Geometry check sheet. Reference: the model listing, model coordinates, mm. Round coordinates to 2 decimals unless told otherwise and drop trailing zeros. Loops run counter-clockwise (first coordinate to the right, second up) from the corner with the lowest first, then second, coordinate; pieces in that order, holes last. Notation, with made-up numbers: (-30.5, 35) -> (-15.5, 35) arc R20 cw to (-15.5, 55) -> close; hole circle Ø3 at (11.25, 6.5). An arc over 180 degrees is marked (long way). Use a Markdown table: item, result. Add a question column.
Q1. Gauge pin test, flat ends, axial feed: P1, Ø3, axis at y = -2, z = 9, coming from the -X side; P2, Ø2, axis at x = -2.5, y = -2.5, coming from the -Z side; P3, Ø1.5, axis at x = -2.5, y = -1, coming from the -Z side. Record the tip position at first contact, or that the pin passes through.
Q2. Sectioned sample at D-D, the plane x = 2.75. Enter the section's corners in (y, z).
Q3. Release check for a two-part mould opening along Z. For faces 1 (the face through (2.76, -2.46, 19.47)), 2 (the face through (0, 0, 19)), 3 (the face through (-1.5, -2.46, 0.07)) record: released by +Z, released by -Z, zero draft, split by the parting line, or undercut.
Q4. Sectioned sample at C-C, the plane z = 1. Enter the section's corners in (x, y), then the cut area to 3 significant figures.
Q5. Sectioned sample at B-B, the plane y = -4. Enter the section's corners in (x, z), then the cut area to 3 significant figures.
Q6. Material ranges on L1, parallel to Z at x = 0, y = -2.75; L2, parallel to Z at x = -1, y = -2.8; L3, parallel to X at y = -4.2, z = 3, recorded low to high.
Q7. Sectioned sample at A-A, the plane x = -0.5. Enter the section's corners in (y, z), then the cut area to 3 significant figures.
```python
from build123d import *

# Parameters (mm, degrees)
F0_R     = 1.5
F1_DEPTH = 5


with BuildPart() as f1:
    # F0 (on Front) → F1 (new body)
    with BuildSketch(Plane.XZ):
        with BuildLine():
            Line((-2, 39.5), (-3.5, 0))
            ThreePointArc((-3.5, 0), (-2.474874, -2.474874), (0, -3.5))
            ThreePointArc((0, -3.5), (2.474874, -2.474874), (3.5, 0))
            Line((3.5, 0), (2, 39.5))
            ThreePointArc((2, 39.5), (1.414214, 40.914214), (0, 41.5))
            ThreePointArc((0, 41.5), (-1.414214, 40.914214), (-2, 39.5))
        make_face()
        Circle(F0_R, mode=Mode.SUBTRACT)
    extrude(amount=F1_DEPTH)


solid = f1.part
```
Values:
| question | item | result |
|---|---|---|
| 1 | P1 | x = -3.22 |
| 1 | P2 | z = -3.16 |
| 1 | P3 | z = -3.03 |
| 2 | outline | (-5, -2.17) -> (0, -2.17) -> (0, 19.75) -> (-5, 19.75) -> close |
| 3 | face 1 | released by +Z |
| 3 | face 2 | zero draft |
| 3 | face 3 | undercut |
| 4 | outline | (-3.46, -5) -> (-1.12, -5) -> (-1.12, 0) -> (-3.46, 0) -> close; (1.12, -5) -> (3.46, -5) -> (3.46, 0) -> (1.12, 0) -> close |
| 4 | area | 23.4 mm^2 |
| 5 | outline | (-3.5, 0) arc R3.5 ccw to (0, -3.5) arc R3.5 ccw to (3.5, 0) -> (2, 39.5) arc R2 ccw to (0, 41.5) arc R2 ccw to (-2, 39.5) -> close; hole circle Ø3 at (0, 0) |
| 5 | area | 236 mm^2 |
| 6 | L1 | -3.5 to -1.5, 1.5 to 41.5 |
| 6 | L2 | -3.35 to -1.12, 1.12 to 41.23 |
| 6 | L3 | -3.39 to 3.39 |
| 7 | outline | (-5, -3.46) -> (0, -3.46) -> (0, -1.41) -> (-5, -1.41) -> close; (-5, 1.41) -> (0, 1.41) -> (0, 41.44) -> (-5, 41.44) -> close |
| 7 | area | 210 mm^2 |
